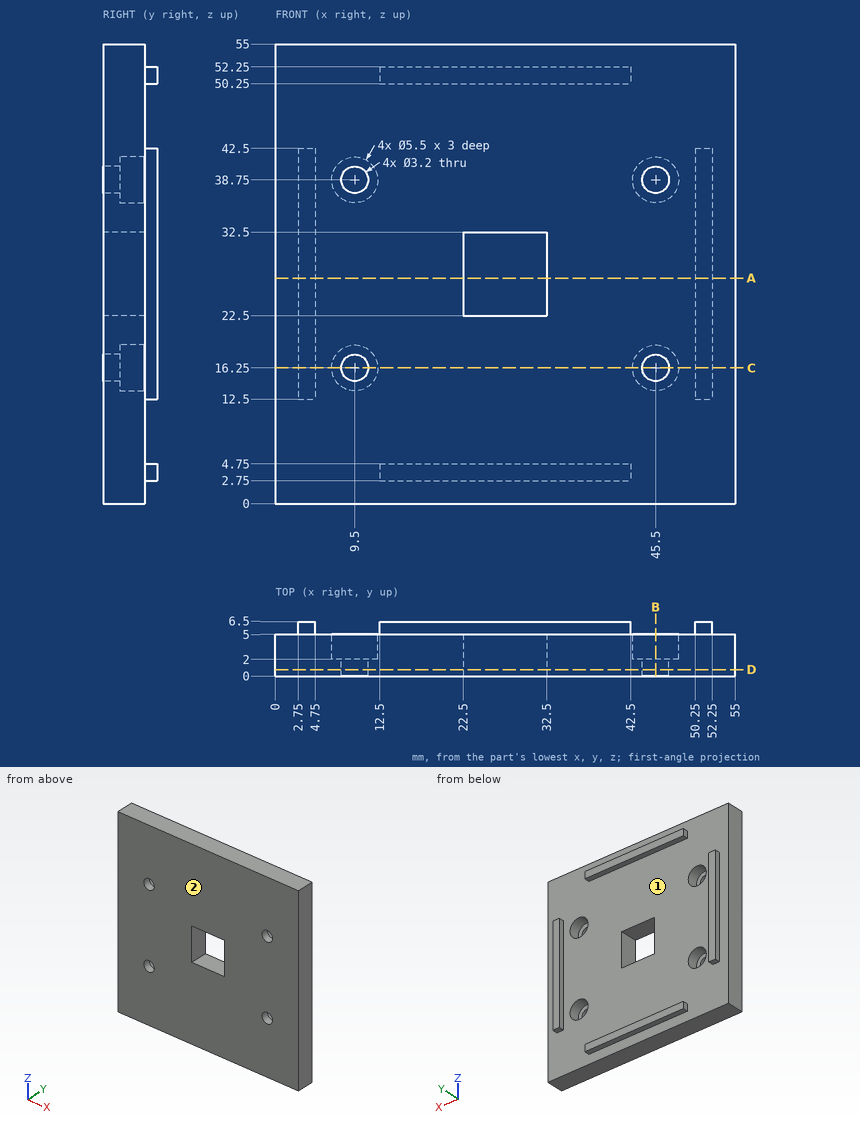
Geometry check sheet. Reference: drawing and pictorial views, mm from the part's lowest x, y, z. Round coordinates to 2 decimals unless told otherwise and drop trailing zeros. Loops run counter-clockwise (first coordinate to the right, second up) from the corner with the lowest first, then second, coordinate; pieces in that order, holes last. Notation, with made-up numbers: (56, 82) -> (108, 82) arc R20 ccw to (108, 102) -> close; hole circle Ø9 at (-14.75, 60.25). An arc over 180 degrees is marked (long way). Answer as a JSON object with one key per item and string values.
Q1. Section check B-B (x = 45.5). Record the boundary of the cut face in (y, z), then the cut area to 3 significant figures.
Data:
{"outline": "(0, 0) -> (5, 0) -> (5, 13.5) -> (2, 13.5) -> (2, 14.65) -> (0, 14.65) -> close; (0, 17.85) -> (2, 17.85) -> (2, 19) -> (5, 19) -> (5, 36) -> (2, 36) -> (2, 37.15) -> (0, 37.15) -> close; (0, 40.35) -> (2, 40.35) -> (2, 41.5) -> (5, 41.5) -> (5, 55) -> (0, 55) -> close", "area": "229 mm2"}
Q2. Go/stop test with flat-tipped pins: P1, Ø3.5, axis at x = 9.5, z = 16.25, coming from the +Y side; P2, Ø1.6, axis at y = 6, z = 51.5, coming from the +X side; P3, Ø3, axis at x = 9.5, z = 38.75, coming from the +Y side; P4, Ø6, axis at x = 26.5, z = 12, coming from the +Y side. Record where each tip stops, or that it passes through.
Data:
{"P1": "stops at y = 2", "P2": "stops at x = 42.5", "P3": "passes through", "P4": "stops at y = 5"}
Q3. Section check D-D (y = 0.75). Record the boundary of the cut face in (x, z), then the cut area to 3 significant figures.
Data:
{"outline": "(0, 0) -> (55, 0) -> (55, 55) -> (0, 55) -> close; hole circle Ø3.2 at (9.5, 16.25); hole circle Ø3.2 at (9.5, 38.75); hole (22.5, 22.5) -> (32.5, 22.5) -> (32.5, 32.5) -> (22.5, 32.5) -> close; hole circle Ø3.2 at (45.5, 16.25); hole circle Ø3.2 at (45.5, 38.75)", "area": "2,890 mm2"}
Q4. Section check C-C (z = 16.25). Record the boundary of the cut face in (x, y), then the cut area to 3 significant figures.
Data:
{"outline": "(0, 0) -> (7.9, 0) -> (7.9, 2) -> (6.75, 2) -> (6.75, 5) -> (4.75, 5) -> (4.75, 6.5) -> (2.75, 6.5) -> (2.75, 5) -> (0, 5) -> close; (11.1, 0) -> (43.9, 0) -> (43.9, 2) -> (42.75, 2) -> (42.75, 5) -> (12.25, 5) -> (12.25, 2) -> (11.1, 2) -> close; (47.1, 0) -> (55, 0) -> (55, 5) -> (52.25, 5) -> (52.25, 6.5) -> (50.25, 6.5) -> (50.25, 5) -> (48.25, 5) -> (48.25, 2) -> (47.1, 2) -> close", "area": "235 mm2"}
Q5. Draft check along X on the marked faces 1 and 2. Enter one of: pulls with the +X half, pulls with the -X half, needs draft (parallel to the pull), parting line crosses it, or undercut.
Data:
{"face 1": "undercut", "face 2": "needs draft"}
Q6. Scan lines: line 1 (X direction, y = 0.9, z = 16.25); line 2 (Z direction, x = 45.5, y = 0.95); line 3 (X direction, y = 2.9, z = 16.25). Record each from-to range of solid material in increasing order. Write a range as from..to.
Data:
{"line 1": "x = 0..7.9, 11.1..43.9, 47.1..55", "line 2": "z = 0..14.65, 17.85..37.15, 40.35..55", "line 3": "x = 0..6.75, 12.25..42.75, 48.25..55"}
Q7. Section check A-A (z = 27). Record the boundary of the cut face in (x, y), then the cut area to 3 significant figures.
Data:
{"outline": "(0, 0) -> (22.5, 0) -> (22.5, 5) -> (4.75, 5) -> (4.75, 6.5) -> (2.75, 6.5) -> (2.75, 5) -> (0, 5) -> close; (32.5, 0) -> (55, 0) -> (55, 5) -> (52.25, 5) -> (52.25, 6.5) -> (50.25, 6.5) -> (50.25, 5) -> (32.5, 5) -> close", "area": "231 mm2"}
